from build123d import *

# Parameters (mm, degrees)
F0_W     = 30
F0_H     = 24
F1_DEPTH = 10
F2_W     = 14
F2_H     = 18
F3_DEPTH = 10.001
F4_R     = 2
F5_R     = 5
F6_SIZE  = 1


with BuildPart() as f1:
    # F0 (on Top) → F1 (new body)
    with BuildSketch(Plane.XY):
        Rectangle(F0_W, F0_H)
    extrude(amount=F1_DEPTH)

    # F2 (on face) → F3 (cut, through all)
    with BuildSketch(Plane.XY.offset(10)):
        with Locations((0, -3)):
            Rectangle(F2_W, F2_H)
    extrude(amount=-F3_DEPTH, mode=Mode.SUBTRACT)

    # F4
    f4_edges = [f1.edges().sort_by_distance(p)[0] for p in [
        (-7, 6, 5),
        (7, 6, 5),
    ]]
    fillet(f4_edges, radius=F4_R)

    # F5
    f5_edges = [f1.edges().sort_by_distance(p)[0] for p in [
        (-15, 12, 5),
        (15, 12, 5),
    ]]
    fillet(f5_edges, radius=F5_R)

    # F6
    f6_edges = [f1.edges().sort_by_distance(p)[0] for p in [
        (0, 12, 10),
    ]]
    chamfer(f6_edges, length=F6_SIZE)


solid = f1.part
Build history of the part. All positions in model axes, mm. A direction names the side the tool comes from. Give positions to 0.01 mm unless a question says otherwise; leave off trailing zeros. Loops run counter-clockwise (first coordinate to the right, second up) from the corner with the lowest first, then second, coordinate; pieces in that order, holes last. Notation, with made-up numbers: (-31.75, 4) - (15.25, 4) arc R26 ccw to (15.25, 37) - close; hole circle Ø2 at (47.25, 15.5). An arc over 180 degrees is marked (long way). Write item = value, one per line. Start each with the question number.
1) Pull direction X, two halves, no side cores. Call faces 3 (the flat face through (0, 7, 10)), 4 (the cylindrical face through (-13, 11, 5)), 5 (the cylindrical face through (-6.43, 5.4, 4.93)): +X half, -X half, draft (parallel to the pull), parting line (faces both ways), or undercut.
2) Band-saw the part on A-A on y = -4. Give the cut face in (x, z), plus the area to 3 significant figures.
3) Tool access for faces 1 (the flat face through (-0.1, 11.5, 9.5)), 2 (the flat face through (0, 6, 5)): list every direction of +Z, -Z, +X, -X, +Y, -Y with a clear straight run to the whole face (end or side of a thin tool).
4) Band-saw the part on C-C on x = 1. Give the cut face in (y, z), plus the area to 3 significant figures.
5) Band-saw the part on B-B on z = 4.75. Give the cut face in (x, y).
6) Probe probe 1 along X at (y, z) = (2.25, 2.25); probe 2 along Y at (x, z) = (2.5, 1.75); probe 3 along X at (y, z) = (4.75, 8.25). List the from-to ranges inside material, lowest first. Write a range as from..to.
7) Drop a flat-ended pin along its axis: pin 1 Ø3 at (y, z) = (9.5, 2.5) entering from -X. Give the stop position or say it passes through.
Final values:
q1.face_3 = draft
q1.face_4 = -X half
q1.face_5 = undercut
q2.outline = (-15, 0) - (-7, 0) - (-7, 10) - (-14, 10) - (-15, 9) - close; (7, 0) - (15, 0) - (15, 9) - (14, 10) - (7, 10) - close
q2.area = 159 mm²
q3.face_1 = +Z, +X, -X, +Y
q3.face_2 = +Z, -Z, -Y
q4.outline = (6, 0) - (12, 0) - (12, 9) - (11, 10) - (6, 10) - close
q4.area = 59.5 mm²
q5.outline = (-15, -12) - (-7, -12) - (-7, 4) arc R2 cw to (-5, 6) - (5, 6) arc R2 cw to (7, 4) - (7, -12) - (15, -12) - (15, 7) arc R5 ccw to (10, 12) - (-10, 12) arc R5 ccw to (-15, 7) - close
q6.probe_1 = -15..-7, 7..15
q6.probe_2 = 6..12
q6.probe_3 = -15..-6.85, 6.85..15
q7.pin_1 = -14.9
